Autodesk Inventor part; units mm, degrees
ref_plane "YZ Plane" through (0, 0, 0) normal (1, 0, 0) x (0, 1, 0)
ref_plane "XZ Plane" through (0, 0, 0) normal (0, 1, 0) x (-1, 0, 0)
ref_plane "XY Plane" through (0, 0, 0) normal (0, 0, 1) x (1, 0, 0)
sketch "Sketch1" plane through (0, 0, 0) normal (1, 0, 0) x (0, 1, 0)
  line L0 (0, 0) -> (0, -10.1)
  line L1 (0, -10.1) -> (5.8, -10.1)
  line L2 (5.8, -10.1) -> (5.8, -12.6)
  line L3 (5.8, -12.6) -> (14.4, -12.6)
  line L4 (14.4, -12.6) -> (14.4, -11.3)
  line L5 (14.4, -11.3) -> (34.4, -11.3)
  line L6 (34.4, -11.3) -> (40.8, -11.3)
  line L7 (40.8, -11.3) -> (40.8, -8.7)
  line L8 (40.8, -8.7) -> (34.4, -11.3)
  line L9 (40.8, -8.7) -> (43.8745, 0)
  line L10 (43.8745, 0) -> (0, 0)
  dimension "d0" = 10.1
  dimension "d1" = 5.8
  dimension "d2" = 90
  dimension "d3" = 2.5
  dimension "d4" = 90
  dimension "d5" = 8.6
  dimension "d6" = 1.3
  dimension "d7" = 90
  dimension "d8" = 20
  dimension "d9" = 6.4
  dimension "d10" = 2.6
revolve "Revolution1" add sketch "Sketch1" angle 360 about axis through (0, 43.8745, 0) along (0, -1, 0) contours L10 L9 L8 L5 L4 L3 L2 L1 L0
properties part number "30_CUBE_openSIM_ObjectiveLens_10x"
The listing builds one solid part. Answer for the finished solid, in the listing's coordinates (mm). A direction names the side the tool comes from. Coordinates: 2 decimals unless noted, no trailing zeros. Loops run counter-clockwise (first coordinate to the right, second up) from the corner with the lowest first, then second, coordinate; pieces in that order, holes last. Notation, with made-up numbers: (73, -37) - (127, -37) arc R26 cw to (127, -21) - close; hole circle Ø6 at (57.5, 56). An arc over 180 degrees is marked (long way). Use a Markdown table: item, result. Add a question column.
1) The part is cut by section B-B, the plane y = 9.5. Give the vertices of the cut face in (x, z).
2) The part is cut by section A-A, the plane y = 21. Give the vertices of the cut face in (x, z).
3) For faces 1 (the flat face through (0, 0, 0)), 2 (the cylindrical face through (-3.39, 24.54, -10.78)), 3 (the flat face through (10.3, 5.8, 0.1)), determine the directions among +Z, -Z, +X, -X, +Y, -Y from which every point of the face is accessible in a straight line to the end or side of a thin tool.
4) Given pin 1 (3 mm diameter, centred on y = 30, z = -5.5, fed in from +X); pin 2 (12 mm diameter, centred on y = 21.5, z = -8, fed in from -X); pin 3 (6 mm diameter, centred on x = -6, y = 20.5, fed in from +Z); pin 4 (7.5 mm diameter, centred on x = 3, z = -1.5, fed in from +Y), each flat-ended and moving along its own axis, determine where each tip first touches the part or whether it passes through.
5) Find the intervals of material crossed by line 1 (Y direction, x = 6.75, z = 9.75); line 2 (X direction, y = 13.5, z = 0.5); line 3 (Y direction, x = -0.25, z = -3.5), in increasing order.
Here are the results:
| question | item | result |
|---|---|---|
| 1 | outline | circle Ø25.2 at (0, 0) |
| 2 | outline | circle Ø22.6 at (0, 0) |
| 3 | face 1 | +Z, -Z, +X, -X, -Y |
| 3 | face 2 | +Y |
| 3 | face 3 | -Y |
| 4 | pin 1 | stops at x = 10.57 |
| 4 | pin 2 | stops at x = -11.12 |
| 4 | pin 3 | stops at z = 10.89 |
| 4 | pin 4 | stops at y = 43.87 |
| 5 | line 1 | y = 5.8 to 14.4 |
| 5 | line 2 | x = -12.59 to 12.59 |
| 5 | line 3 | y = 0 to 42.63 |
